```python
from build123d import *

# Parameters (mm, degrees)
F0_W           = 635
F0_H           = 25.4
F1_DEPTH       = 25.4
F3_D           = 6.35
F3_CBORE_D     = 12.7
F3_CBORE_DEPTH = 6.35
F4_W           = 0.5842
F4_H           = 25.4
F5_DEPTH       = 19.05
F6_W           = 3.175
F6_H           = 25.4
F7_DEPTH       = 12.7


with BuildPart() as f1:
    # F0 (on Top) → F1 (new body)
    with BuildSketch(Plane.XY):
        Rectangle(F0_W, F0_H)
    extrude(amount=F1_DEPTH)

    # F3 (through all)
    with Locations(Plane.XY.offset(25.4)):
        with Locations((-285.75, 0), (285.75, 0)):
            CounterBoreHole(F3_D / 2, F3_CBORE_D / 2, F3_CBORE_DEPTH)

    # F4 (on face) → F5 (cut)
    with BuildSketch(Plane.XY.offset(25.4)):
        with Locations((25.4, 0)):
            Rectangle(F4_W, F4_H)
    extrude(amount=-F5_DEPTH, mode=Mode.SUBTRACT)

    # F6 (on face) → F7 (cut)
    with BuildSketch(Plane.XY.offset(25.4)):
        with Locations((25.4, 0)):
            Rectangle(F6_W, F6_H)
    extrude(amount=-F7_DEPTH, mode=Mode.SUBTRACT)


solid = f1.part
```
Verification items for the finished model (mm, model axes). A direction names the side the tool comes from. Coordinates: 2 decimals unless noted, no trailing zeros. Answer as a JSON object with one key per item and string values. Group by question number.
(1) Material ranges on line 1 (X direction, y = 0.75, z = 14.5); line 2 (Y direction, x = -285.75, z = 7) (3 decimals); line 3 (X direction, y = -1.25, z = 19.25), recorded low to high.
(2) Tool access check on faces 1 (the face through (-317.5, 0, 13)), 2 (the face through (-289, -1, 19.05)). Record the directions out of +Z, -Z, +X, -X, +Y, -Y that give a thin tool (end or side, any length) a straight path to the whole face; none if there is none.
(3) Release check for a two-part mould opening along X. For faces 3 (the face through (26.987, 0, 19)), 4 (the face through (23.812, 0, 19)), 5 (the face through (317.5, 0, 13)), 6 (the face through (170, 0, 25.4)) record: +X half, -X half, draft (parallel to the pull), parting line (faces both ways), or undercut.
(4) Gauge pin test, flat ends, axial feed: pin 1 (6.5 mm diameter, centred on x = -288.5, y = -0.5, fed in from +Z); pin 2 (0.6 mm diameter, centred on x = 24.5, y = 4, fed in from +Z). Record the tip position at first contact, or that the pin passes through.
Reply:
{
 "1": {"line 1": "-317.5 to -288.84, -282.66 to 23.81, 26.99 to 282.66, 288.84 to 317.5", "line 2": "-12.7 to -3.175, 3.175 to 12.7", "line 3": "-317.5 to -291.98, -279.52 to 23.81, 26.99 to 279.52, 291.98 to 317.5"},
 "2": {"face 1": "+Z, -Z, -X, +Y, -Y", "face 2": "+Z"},
 "3": {"face 3": "undercut", "face 4": "undercut", "face 5": "+X half", "face 6": "draft"},
 "4": {"pin 1": "z = 19.05", "pin 2": "z = 12.7"}
}
